The model under review builds one solid part; all positions refer to its coordinate system, in mm. A direction names the side the tool comes from. Coordinates: 2 decimals unless noted, no trailing zeros. Write each loop counter-clockwise with the first axis right and the second up, starting at its lowest first coordinate (ties: lowest second). Pieces come first, ordered by that corner, then holes.
Autodesk Inventor part; units mm, degrees
ref_plane "YZ Plane" through (0, 0, 0) normal (1, 0, 0) x (0, 1, 0)
ref_plane "XZ Plane" through (0, 0, 0) normal (0, 1, 0) x (-1, 0, 0)
ref_plane "XY Plane" through (0, 0, 0) normal (0, 0, 1) x (1, 0, 0)
sketch "Sketch1" plane through (0, 0, 0) normal (0, 0, 1) x (1, 0, 0)
  line L0 (0, 0) -> (140, 0)
  line L1 (140, 0) -> (140, 80)
  line L2 (140, 80) -> (0, 80)
  line L3 (0, 80) -> (0, 0)
  dimension "d0" = 140
  dimension "d1" = 80
extrude "Extrusion1" add sketch "Sketch1" along normal blind 2
sketch "Sketch2" plane through (0, 0, 2) normal (0, 0, 1) x (1, 0, 0)
  line L0 (0, 80) -> (2, 80)
  line L1 (2, 80) -> (2, 78)
  line L2 (2, 78) -> (0, 78)
  line L3 (0, 78) -> (0, 80)
  line L4 (2, 78) -> (138, 78)
  line L5 (138, 78) -> (138, 2)
  line L6 (138, 2) -> (2, 2)
  line L7 (2, 2) -> (2, 78)
  dimension "d4" = 2
  dimension "d5" = 2
  dimension "d6" = 136
  dimension "d7" = 76
extrude "Extrusion2" add sketch "Sketch2" along normal blind 3 contours L4 L5 L6 L7
sketch "Sketch3" plane through (0, 0, 2) normal (0, 0, 1) x (1, 0, 0)
  line L0 (0, 0) -> (140, 0)
  line L1 (2, 2) -> (138, 2)
  line L2 (138, 2) -> (138, 0)
  line L3 (138, 0) -> (2, 0)
  line L4 (2, 0) -> (2, 2)
extrude "Extrusion3" add sketch "Sketch3" along normal blind 3
sketch "Sketch4" plane through (0, 0, 0) normal (0, 0, -1) x (-1, 0, 0)
  line L0 (0, 0) -> (-140, 0)
  line L1 (0, 80) -> (0, 0)
  line L2 (-140, 0) -> (0, 0)
  line L3 (0, 0) -> (0, 1)
  line L4 (0, 1) -> (-140, 1)
  line L5 (-140, 1) -> (-140, 0)
  dimension "d12" = 1
extrude "Extrusion4" cut sketch "Sketch4" against normal blind 7.5
sketch "Sketch5" plane through (0, 0, 0) normal (0, 0, -1) x (-1, 0, 0)
  line L0 (-140, 80) -> (0, 80)
  line L1 (0, 80) -> (0, 81)
  line L2 (0, 81) -> (-140, 81)
  line L3 (-140, 81) -> (-140, 80)
  point P0 (0, 0)
  dimension "d15" = 1
extrude "Extrusion5" add sketch "Sketch5" against normal blind 2
sketch "Sketch6" plane through (0, 0, 5) normal (0, 0, 1) x (1, 0, 0)
  line L0 (138, 78) -> (2, 78)
  line L1 (2, 1) -> (3, 1)
  line L2 (3, 1) -> (3, 78)
  line L3 (3, 78) -> (2, 78)
  line L4 (2, 78) -> (2, 1)
  line L5 (138, 1) -> (137, 1)
  line L6 (137, 1) -> (137, 78)
  line L7 (137, 78) -> (138, 78)
  line L8 (138, 78) -> (138, 1)
  point P0 (0, 0)
  dimension "d18" = 1
  dimension "d19" = 1
extrude "Extrusion6" cut sketch "Sketch6" against normal blind 3
sketch "Sketch7" plane through (0, 0, 0) normal (0, 0, -1) x (-1, 0, 0)
  line L0 (-140, 1) -> (0, 1)
  line L1 (0, 1) -> (0, 81)
  line L2 (0, 81) -> (-140, 81)
  line L3 (-140, 1) -> (-140, 81)
  line L4 (0, 1) -> (-165, 1)
  line L5 (-165, 1) -> (-165, 81)
  line L6 (-165, 81) -> (0, 81)
  line L7 (0, 81) -> (0, 1)
  point P0 (0, 0)
  dimension "d22" = 165
extrude "Extrusion7" add sketch "Sketch7" against normal blind 2 contours L4 L5 L6 L3
sketch "Sketch9" plane through (0, 0, 2) normal (0, 0, 1) x (1, 0, 0)
  line L0 (137, 1) -> (162, 1)
  line L1 (162, 1) -> (162, 78)
  line L2 (162, 78) -> (137, 78)
  line L3 (137, 78) -> (137, 1)
  point P0 (0, 0)
  dimension "d25" = 25
extrude "Extrusion8" add sketch "Sketch9" along normal blind 3
sketch "Sketch10" plane through (0, 0, 0) normal (0, 0, -1) x (-1, 0, 0)
  line L0 (0, 1) -> (-10, 1)
  line L1 (-10, 1) -> (-10, 11)
  line L2 (-10, 11) -> (0, 11)
  line L3 (0, 11) -> (0, 1)
  line L4 (0, 81) -> (-10, 81)
  line L5 (-10, 81) -> (-10, 71)
  line L6 (-10, 71) -> (0, 71)
  line L7 (0, 71) -> (0, 81)
  line L8 (-10, 71) -> (-55, 71)
  line L9 (-55, 71) -> (-55, 11)
  line L10 (-55, 11) -> (-10, 11)
  line L11 (-10, 11) -> (-10, 71)
  point P0 (0, 0)
  dimension "d28" = 10
  dimension "d29" = 10
  dimension "d30" = 10
  dimension "d31" = 10
  dimension "d32" = 45
extrude "Extrusion9" cut sketch "Sketch10" against normal blind 10.25 contours L10 L9 L8 L11
properties part number "Receiver Case top"
Item 1: Take a section at B-B, the plane y = 46.5. Write out the cut boundary in (x, z), plus the area to 3 significant figures.
Solved:
outline: (0, 0) - (10, 0) - (10, 5) - (3, 5) - (3, 2) - (0, 2) - close; (55, 0) - (165, 0) - (165, 2) - (162, 2) - (162, 5) - (55, 5) - close
area: 582 mm2
Item 2: For pin 1 (1.5 mm diameter, centred on y = 31.5, z = 3, fed in from +X); pin 2 (1 mm diameter, centred on y = 15.5, z = 3, fed in from -X), all flat-tipped, find the tip position at first contact; note any pin that passes through.
Solved:
pin 1: stops at x = 162
pin 2: stops at x = 3
Item 3: Machinability: for faces 4 (the face through (84, 78, 3)), 5 (the face through (102, 42, 0)), 6 (the face through (10, 41, 2)), 7 (the face through (3, 39, 4)), 8 (the face through (99, 40, 5)), which of the approach directions +Z, -Z, +X, -X, +Y, -Y give a long, thin tool a straight path to every point of the face, cutting with its end or side? Answer none if there is none.
Solved:
face 4: +Z, +X, -X, +Y
face 5: -Z, +X, -X, +Y, -Y
face 6: +Z, -Z
face 7: +Z, -X, +Y, -Y
face 8: +Z, +X, -X, +Y, -Y
Item 4: Take a section at A-A, the plane x = 35.5. Write out the cut boundary in (y, z).
Solved:
outline: (1, 0) - (11, 0) - (11, 5) - (1, 5) - close; (71, 0) - (81, 0) - (81, 2) - (78, 2) - (78, 5) - (71, 5) - close
Item 5: To check wall thickness, follow line 1 along Y through (x, z) = (14.5, 4.55); line 2 along X through (y, z) = (27, 0.35); line 3 along X through (y, z) = (40, 3.05). State the ranges of each line that lie inside material, in increasing order.
Solved:
line 1: y = 1 to 11, 71 to 78
line 2: x = 0 to 10, 55 to 165
line 3: x = 3 to 10, 55 to 162
Item 6: Take a section at D-D, the plane y = 7.5. Write out the cut boundary in (x, z).
Solved:
outline: (0, 0) - (165, 0) - (165, 2) - (162, 2) - (162, 5) - (3, 5) - (3, 2) - (0, 2) - close
Item 7: Take a section at C-C, the plane z = 0.75. Write out the cut boundary in (x, y), plus the area to 3 significant figures.
Solved:
outline: (0, 1) - (165, 1) - (165, 81) - (0, 81) - close; hole (10, 11) - (55, 11) - (55, 71) - (10, 71) - close
area: 10,500 mm2
Item 8: Mouldability with a two-part tool opening along X and no side actions: class faces 1 (the face through (81, 1, 2)), 2 (the face through (55, 41, 2)), 3 (the face through (162, 39, 3)) as pulls with the +X half, pulls with the -X half, needs draft (parallel to the pull), parting line crosses it, or undercut.
Solved:
face 1: needs draft
face 2: undercut
face 3: pulls with the +X half
